Could you check a few things on this model? Use its own coordinates, in mm. A direction names the side the tool comes from. Give positions to 0.01 mm unless a question says otherwise; leave off trailing zeros. Write each loop counter-clockwise with the first axis right and the second up, starting at its lowest first coordinate (ties: lowest second). Pieces come first, ordered by that corner, then holes. Notation, with made-up numbers: (63, 72.25) - (108, 72.25) arc R10 ccw to (108, 86.25) - close; hole circle Ø8 at (53, -20). An arc over 180 degrees is marked (long way). Answer as CSV lines item,"result". Start each with the question number.
Q1. Imagine slicing it at D-D on x = 1.2. List the corners of the cut face in (y, z) for me, and give its area (3 significant figures).
Q2. Will these pins go through, and if not, where does the flat tip stop? pin 1 Ø2.5 at (y, z) = (0.5, 3) entering from -X; pin 2 Ø1 at (x, z) = (2, 3.5) entering from -Y.
Q3. Imagine slicing it at C-C on y = 1.5. List the corners of the cut face in (x, z) for me, and give its area (3 significant figures).
Q4. We'd pull the mould along Z, two halves only. Please class faces 3 (the face through (-2, -3, 3)), 4 (the face through (-2.01, 0.35, 1.69)), 5 (the face through (0, 0, 6.5)): pulls with the +Z half, pulls with the -Z half, needs draft (parallel to the pull), parting line crosses it, or undercut.
Q5. If I drill on line 1 along Z through (x, y) = (-2.2, 0); line 2 along X through (y, z) = (-2.25, 1.75); line 3 along X through (y, z) = (-1.5, 4), over which ranges is the centre line in solid material (lowest first)?
Q6. On a 3-axis mill with a long thin cutter (end or side, diameter ignored), from which of +Z, -Z, +X, -X, +Y, -Y can I reach the whole of each face in a straight line? I mean faces 1 (the face through (2.1, -2.14, 3.3)), 2 (the face through (-1, 0, 3)). Say none if no direction works.
Q7. Imagine slicing it at B-B on x = -2.5. List the corners of the cut face in (y, z) for me, and give its area (3 significant figures).
```python
from build123d import *

# Parameters (mm, degrees)
SKETCH1_W           = 6
SKETCH1_H           = 6
BOSS_EXTRUDE1_DEPTH = 6.5
FILLET1_R           = 3
SKETCH2_R           = 1.6
CUT_EXTRUDE1_DEPTH  = 2


with BuildPart() as part:
    # Sketch1 → Boss-Extrude1 (new body)
    with BuildSketch(Plane.XY):
        Rectangle(SKETCH1_W, SKETCH1_H)
    extrude(amount=BOSS_EXTRUDE1_DEPTH)

    # Fillet1
    fillet1_edges = [part.edges().sort_by_distance(p)[0] for p in [
        (3, -3, 3.25),
        (3, 3, 3.25),
    ]]
    fillet(fillet1_edges, radius=FILLET1_R - 0.0001)  # a hair under: the kernel refuses the full size

    # Sketch2 → Cut-Extrude1 (cut)
    with BuildSketch(Plane.ZY.offset(3)):
        with Locations(Location((3.25, 0, 0), (0, 0, 270))):
            Circle(SKETCH2_R)
    extrude(amount=-CUT_EXTRUDE1_DEPTH, mode=Mode.SUBTRACT)


solid = part.part
```
Conclusion:
1,outline,"(-2.75, 0) - (2.75, 0) - (2.75, 6.5) - (-2.75, 6.5) - close"
1,area,"35.7 mm^2"
2,pin 1,"x = -3"
2,pin 2,"y = -2.6"
3,outline,"(-3, 0) - (2.6, 0) - (2.6, 6.5) - (-3, 6.5) - (-3, 3.81) - (-1, 3.81) - (-1, 2.69) - (-3, 2.69) - close"
3,area,"34.2 mm^2"
4,face 3,"needs draft"
4,face 4,"undercut"
4,face 5,"pulls with the +Z half"
5,line 1,"0 to 1.65, 4.85 to 6.5"
5,line 2,"-3 to 1.98"
5,line 3,"-3 to 2.6"
6,face 1,"+Z, -Z, +X, -Y"
6,face 2,"-X"
7,outline,"(-3, 0) - (3, 0) - (3, 6.5) - (-3, 6.5) - close; hole circle Ø3.2 at (0, 3.25)"
7,area,"31.0 mm^2"
